The listing builds one solid part. Answer for the finished solid, in the listing's coordinates (mm). Give positions to 0.01 mm unless a question says otherwise; leave off trailing zeros. Order: outer loops, then holes, each group sorted by start corner. A loop starts at its lowest first (then second) coordinate and runs counter-clockwise, first axis right, second up.
```python
from build123d import *

# Parameters (mm, degrees)
SKETCH1_W           = 25.3
SKETCH1_H           = 25.3
SKETCH1_R           = 2.15
SKETCH1_R_2         = 3.45
BOSS_EXTRUDE1_DEPTH = 3
FILLET1_R           = 2


with BuildPart() as part:
    # Sketch1 → Boss-Extrude1 (new body)
    with BuildSketch(Plane(origin=(0, 0, 0), x_dir=(1, 0, 0), z_dir=(0, 1, 0))):
        with Locations((12.65, 12.65)):
            Rectangle(SKETCH1_W, SKETCH1_H)
        with Locations((4.65, 4.65)):
            Circle(SKETCH1_R, mode=Mode.SUBTRACT)
        with Locations((12.65, 4.65)):
            Circle(SKETCH1_R, mode=Mode.SUBTRACT)
        with Locations((20.65, 4.65)):
            Circle(SKETCH1_R, mode=Mode.SUBTRACT)
        with Locations((4.65, 12.65)):
            Circle(SKETCH1_R, mode=Mode.SUBTRACT)
        with Locations((4.65, 20.65)):
            Circle(SKETCH1_R, mode=Mode.SUBTRACT)
        with Locations((20.65, 12.65)):
            Circle(SKETCH1_R, mode=Mode.SUBTRACT)
        with Locations((20.65, 20.65)):
            Circle(SKETCH1_R, mode=Mode.SUBTRACT)
        with Locations((12.65, 20.65)):
            Circle(SKETCH1_R, mode=Mode.SUBTRACT)
        with Locations((12.65, 12.65)):
            Circle(SKETCH1_R_2, mode=Mode.SUBTRACT)
    extrude(amount=BOSS_EXTRUDE1_DEPTH)

    # Fillet1
    fillet1_edges = [part.edges().sort_by_distance(p)[0] for p in [
        (0, 1.5, -25.3),
        (25.3, 1.5, -25.3),
        (25.3, 1.5, 0),
        (0, 1.5, 0),
    ]]
    fillet(fillet1_edges, radius=FILLET1_R)


solid = part.part
```
1) Straight lines are drawn through the part: probe 1 along X at (y, z) = (2.95, -4.75); probe 2 along Z at (x, y) = (4.65, 1.7); probe 3 along X at (y, z) = (1.25, -12.5). For each, find the intervals that lie inside material, in ascending order.
Geometry says:
probe 1: x = 0 to 2.5, 6.8 to 10.5, 14.8 to 18.5, 22.8 to 25.3
probe 2: z = -25.3 to -22.8, -18.5 to -14.8, -10.5 to -6.8, -2.5 to 0
probe 3: x = 0 to 2.51, 6.79 to 9.2, 16.1 to 18.51, 22.79 to 25.3
2) Find section D-D (x = 15.5). Write down the section's boundary in (y, z).
Geometry says:
outline: (0, -25.3) - (3, -25.3) - (3, -14.59) - (0, -14.59) - close; (0, -10.71) - (3, -10.71) - (3, 0) - (0, 0) - close
3) Find section C-C (y = 1.9). Count the separate pieces of the cut face and the enclosed holes in it, then the cut area to 3 significant figures.
Geometry says:
separate pieces: 1
enclosed holes: 9
area: 483 mm2
4) Find section B-B (z = -4.65). Write down the section's boundary in (x, y).
Geometry says:
outline: (0, 0) - (2.5, 0) - (2.5, 3) - (0, 3) - close; (6.8, 0) - (10.5, 0) - (10.5, 3) - (6.8, 3) - close; (14.8, 0) - (18.5, 0) - (18.5, 3) - (14.8, 3) - close; (22.8, 0) - (25.3, 0) - (25.3, 3) - (22.8, 3) - close
5) For a pull along X with two mould halves and no side action, classify faces 1 (the flat face through (13, 1, -25.3)), 2 (the cylindrical face through (0.57, 1.52, -24.7)), 3 (the cylindrical face through (18.5, 1.5, -4.7)) as +X half, -X half, draft (parallel to the pull), parting line (faces both ways), or undercut.
Geometry says:
face 1: draft
face 2: -X half
face 3: undercut
6) Given P1, Ø2.5, axis at x = 4.65, z = -4.65, coming from the -Y side, flat-ended and moving along its own axis, determine where the tip first touches the part or whether it passes through.
Geometry says:
P1: passes through
7) Find section A-A (x = 20.65). Write down the section's boundary in (y, z), then the cut area to 3 significant figures.
Geometry says:
outline: (0, -25.3) - (3, -25.3) - (3, -22.8) - (0, -22.8) - close; (0, -18.5) - (3, -18.5) - (3, -14.8) - (0, -14.8) - close; (0, -10.5) - (3, -10.5) - (3, -6.8) - (0, -6.8) - close; (0, -2.5) - (3, -2.5) - (3, 0) - (0, 0) - close
area: 37.2 mm2
